Read the model definition and answer for the solid it produces. Units are mm, in the model's axes. Face numbers are marked on the shaded views. A direction names the side the tool comes from. Coordinates: 2 decimals unless noted, no trailing zeros. Order: outer loops, then holes, each group sorted by start corner. A loop starts at its lowest first (then second) coordinate and runs counter-clockwise, first axis right, second up. Notation, with made-up numbers: (68, -26.75) - (92, -26.75) arc R14 ccw to (92, -2.75) - close; hole circle Ø8 at (-38.75, 6.5). An arc over 180 degrees is marked (long way). Use one line per item in the form item = value.
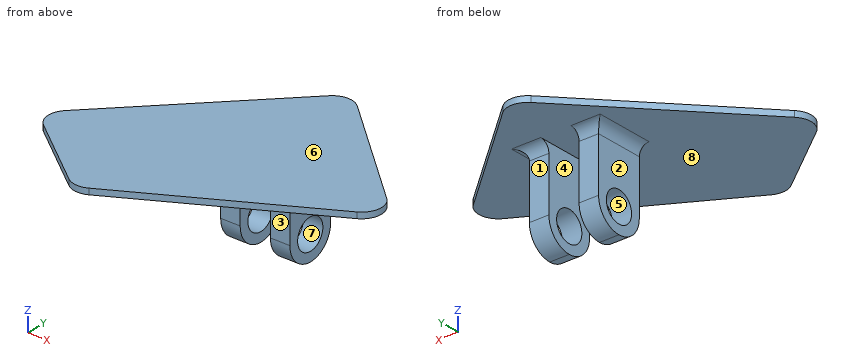
Autodesk Inventor part; units mm, degrees
ref_plane "YZ Plane" through (0, 0, 0) normal (1, 0, 0) x (0, 1, 0)
ref_plane "XZ Plane" through (0, 0, 0) normal (0, 1, 0) x (-1, 0, 0)
ref_plane "XY Plane" through (0, 0, 0) normal (0, 0, 1) x (1, 0, 0)
sketch "Sketch1" plane through (0, 0, 0) normal (0, 0, 1) x (1, 0, 0)
  line L0 (22.1506, 55.679) -> (98.2363, -11.7464)
  line L1 (98.2363, -11.7464) -> (-13.4178, -74.2233)
  line L2 (-13.4178, -74.2233) -> (-63.8323, -35.4735)
  line L3 (-63.8323, -35.4735) -> (22.1506, 55.679)
  point P0 (0, 0)
extrude "Extrusion1" add sketch "Sketch1" along normal blind 3
fillet "Fillet1" radius 10 4 edges at (98.2363, -11.7464, 1.5) (-13.4178, -74.2233, 1.5) (22.1506, 55.679, 1.5) (-63.8323, -35.4735, 1.5)
sketch "Sketch2" plane through (0, 0, 0) normal (0, 0, -1) x (-1, 0, 0)
  line L0 (-41.2625, -6.2798) -> (-5.7625, -6.2798)
  line L1 (-5.7625, -6.2798) -> (-5.7625, 18.7202)
  line L2 (-5.7625, 18.7202) -> (-41.2625, 18.7202)
  line L3 (-41.2625, 18.7202) -> (-41.2625, -6.2798)
  line L4 (-41.2625, -6.2798) -> (-5.7625, 18.7202) construction
  line L5 (-5.7625, -6.2798) -> (-41.2625, 18.7202) construction
  line L6 (-31.2625, -6.2798) -> (-15.7625, -6.2798)
  line L7 (-15.7625, -6.2798) -> (-15.7625, 18.7202)
  line L8 (-15.7625, 18.7202) -> (-31.2625, 18.7202)
  line L9 (-31.2625, 18.7202) -> (-31.2625, -6.2798)
  line L10 (-31.2625, -6.2798) -> (-15.7625, 18.7202) construction
  line L11 (-15.7625, -6.2798) -> (-31.2625, 18.7202) construction
  point P0 (0, 0)
  point P1 (-23.5125, 6.2202)
  point P2 (-31.2625, -6.2798)
  point P3 (-15.7625, -6.2798)
  dimension "d3" = 10
  dimension "d4" = 25
  dimension "d8" = 15.5
extrude "Extrusion2" add sketch "Sketch2" along normal blind 45 contours L3 L2 L9 L0 | L7 L2 L1 L0
fillet "Fillet2" radius 12.5 4 edges at (10.7625, 18.7202, -45) (36.2625, 18.7202, -45) (10.7625, -6.2798, -45) (36.2625, -6.2798, -45)
sketch "Sketch3" plane through (5.7625, -6.2798, 0) normal (-1, 0, 0) x (0, 0, 1)
  arc A0 (-32.5, 25) -> (-32.5, 0) centre (-32.5, 12.5) ccw
  circle A1 centre (-32.5, 12.5) radius 7.75
  point P0 (0, 6.2798)
  dimension "d9" = 15.5
extrude "Extrusion3" cut sketch "Sketch3" against normal up to surface (35.5 mm away)
fillet "Fillet3" radius 5 4 edges at (5.7625, 6.2202, 0) (10.7625, 18.7202, 0) (41.2625, 6.2202, 0) (36.2625, 18.7202, 0)
properties part number "Upper Back Plate"
(1) The mould has two halves that part along Z. Classify the marked faces 5, 6, 7 and 8: +Z half, -Z half, draft (parallel to the pull), parting line (faces both ways), or undercut.
Answer list:
face_5 = undercut
face_6 = +Z half
face_7 = undercut
face_8 = -Z half
(2) Section A-A, the plane z = -11 is taken. Write down the section's boundary in (x, y), then the cut area to 3 significant figures.
Answer list:
outline = (5.76, -6.28) - (15.76, -6.28) - (15.76, 18.72) - (5.76, 18.72) - close; (31.26, -6.28) - (41.26, -6.28) - (41.26, 18.72) - (31.26, 18.72) - close
area = 500 mm2
(3) Section C-C, the plane y = -59 is taken. Write down the section's boundary in (x, z).
Answer list:
outline = (-33.22, 0) - (13.79, 0) - (13.79, 3) - (-33.22, 3) - close
(4) Straight lines are drawn through the part: L1, parallel to X at y = -1, z = -37; L2, parallel to Y at x = 10, z = -32; L3, parallel to Z at x = 19.5, y = -1.5. For each, find the intervals that lie inside material, in ascending order.
Answer list:
L1 = 5.76 to 15.76, 31.26 to 41.26
L2 = -6.28 to -1.51, 13.95 to 18.72
L3 = 0 to 3
(5) Which of the six approach directions +Z, -Z, +X, -X, +Y, -Y give full straight-line access (tool end or side, diameter ignored) to the marked faces 1, 2, 3 and 4?
Answer list:
face_1 = -Z, +X, -X, +Y
face_2 = -Z, -X, +Y, -Y
face_3 = -Z, +X, -X, -Y
face_4 = -Z, +Y, -Y
(6) Section B-B, the plane x = -34 is taken. Write down the section's boundary in (y, z), then the cut area to 3 significant figures.
Answer list:
outline = (-58.4, 0) - (-3.85, 0) - (-3.85, 3) - (-58.4, 3) - close
area = 164 mm2
(7) Given pin 1 Ø8 at (x, z) = (11, -17.5) entering from +Y; pin 2 Ø12.5 at (y, z) = (6.5, -22.5) entering from -X; pin 3 Ø7.5 at (x, z) = (5.5, -12.5) entering from -Y, each flat-ended and moving along its own axis, determine where each tip first touches the part or whether it passes through.
Answer list:
pin_1 = 18.72
pin_2 = 5.76
pin_3 = -6.28
